The drawing under review shows one solid part. Ordinate dimensions are in mm from its lowest x, y, z. A direction names the side the tool comes from. Give positions to 0.01 mm unless a question says otherwise; leave off trailing zeros. Order: outer loops, then holes, each group sorted by start corner. A loop starts at its lowest first (then second) coordinate and runs counter-clockwise, first axis right, second up. Notation, with made-up numbers: (31.5, -38) -> (59.5, -38) arc R11 ccw to (59.5, -28) -> close; hole circle Ø9 at (1.5, -38). An arc over 180 degrees is marked (long way). One line per item, written item: value.
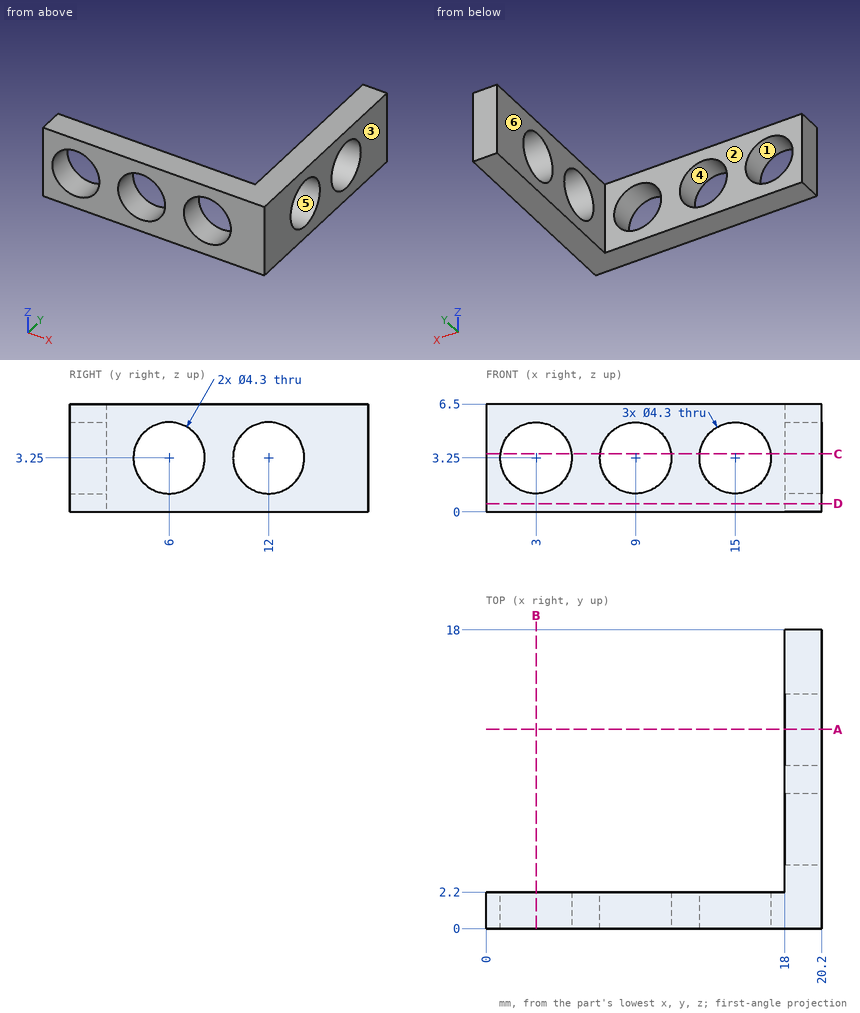
Item 1: To check wall thickness, follow line 1 along Y through (x, z) = (18.8, 3.25); line 2 along Z through (x, y) = (9, 0.7); line 3 along X through (y, z) = (3.25, 4). State the ranges of each line that lie inside material, in increasing order. Write a range as from..to.
Returned:
line 1: 0..3.85, 8.15..9.85, 14.15..18
line 2: 0..1.1, 5.4..6.5
line 3: 18..20.2
Item 2: Add section D-D on z = 0.5. Give the boundary of the cut face in (x, y), plus the area to 3 significant figures.
Returned:
outline: (0, 0) -> (20.2, 0) -> (20.2, 18) -> (18, 18) -> (18, 2.2) -> (0, 2.2) -> close
area: 79.2 mm²
Item 3: Draft analysis for pull direction X (two halves, no side actions). For the marked faces 1, 2, 3 and 4, state which applies: pulls with the +X half, pulls with the -X half, needs draft (parallel to the pull), parting line crosses it, or undercut.
Returned:
face 1: undercut
face 2: needs draft
face 3: pulls with the +X half
face 4: undercut
Item 4: Add section C-C on z = 3.5. Give the boundary of the cut face in (x, y).
Returned:
outline: (0, 0) -> (0.86, 0) -> (0.86, 2.2) -> (0, 2.2) -> close; (5.14, 0) -> (6.86, 0) -> (6.86, 2.2) -> (5.14, 2.2) -> close; (11.14, 0) -> (12.86, 0) -> (12.86, 2.2) -> (11.14, 2.2) -> close; (17.14, 0) -> (20.2, 0) -> (20.2, 3.86) -> (18, 3.86) -> (18, 2.2) -> (17.14, 2.2) -> close; (18, 8.14) -> (20.2, 8.14) -> (20.2, 9.86) -> (18, 9.86) -> close; (18, 14.14) -> (20.2, 14.14) -> (20.2, 18) -> (18, 18) -> close
Item 5: Machinability: for the marked faces 5 and 6, which of the approach directions +Z, -Z, +X, -X, +Y, -Y give a long, thin tool a straight path to every point of the face, cutting with its end or side? Answer none if there is none.
Returned:
face 5: +X, -X
face 6: +Z, -Z, -X, +Y
Item 6: Add section B-B on x = 3. Give the boundary of the cut face in (y, z).
Returned:
outline: (0, 0) -> (2.2, 0) -> (2.2, 1.1) -> (0, 1.1) -> close; (0, 5.4) -> (2.2, 5.4) -> (2.2, 6.5) -> (0, 6.5) -> close
Item 7: Add section A-A on y = 12. Give the boundary of the cut face in (x, z), plus the area to 3 significant figures.
Returned:
outline: (18, 0) -> (20.2, 0) -> (20.2, 1.1) -> (18, 1.1) -> close; (18, 5.4) -> (20.2, 5.4) -> (20.2, 6.5) -> (18, 6.5) -> close
area: 4.84 mm²
Item 8: Clearance check with flat-ended pins moving along their axes: P1, Ø1, axis at y = 8, z = 3, coming from the -X side; P2, Ø3, axis at x = 4.5, z = 1.5, coming from the +Y side; P3, Ø6, axis at x = 12.5, y = 14, coming from the +Z side. State where each tip first meets the part, or that it passes through.
Returned:
P1: x = 18
P2: y = 2.2
P3: through
